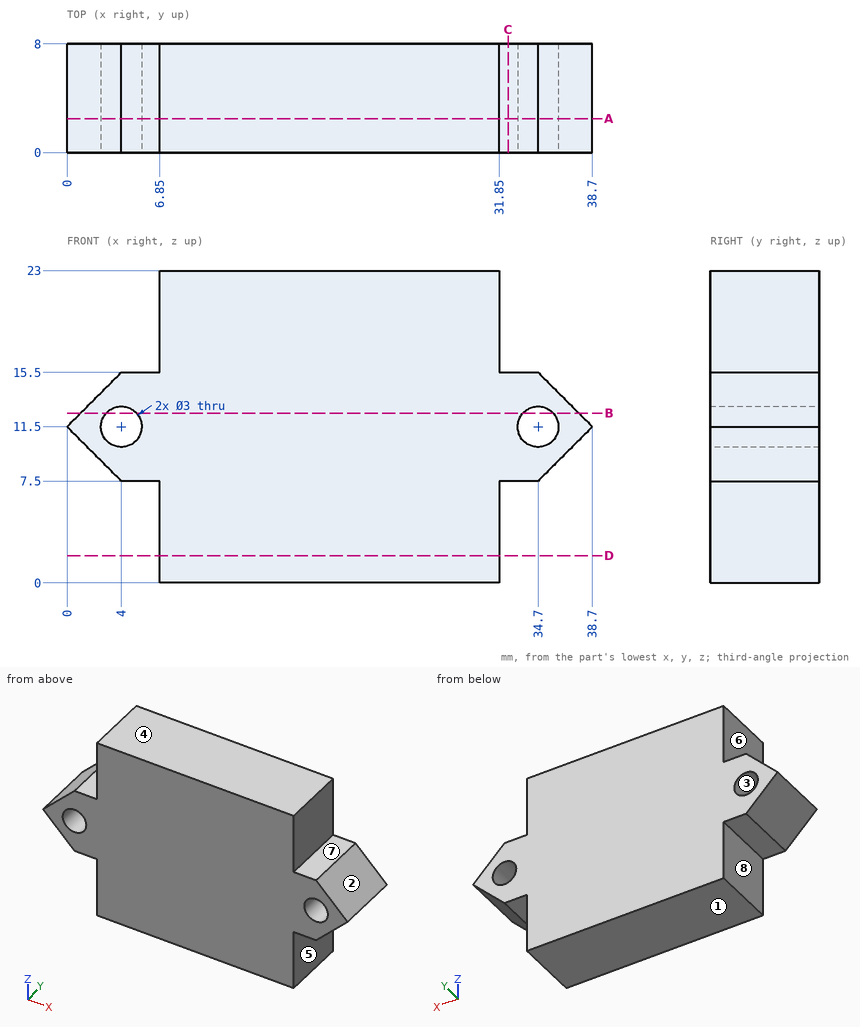
Verification items for this drawing (mm, ordinates from the low corner). A direction names the side the tool comes from. Coordinates: 2 decimals unless noted, no trailing zeros. Loops run counter-clockwise (first coordinate to the right, second up) from the corner with the lowest first, then second, coordinate; pieces in that order, holes last. Notation, with made-up numbers: (-12, 53) -> (37, 53) arc R34 cw to (37, 88) -> close; hole circle Ø8 at (2.25, 11.25). An arc over 180 degrees is marked (long way). Answer in a Markdown table with one row per item. Add a question column.
1. Section check C-C, the plane x = 32.5. Enter the section's corners in (y, z).
2. Section check D-D, the plane z = 2. Enter the section's corners in (x, y), then the cut area to 3 significant figures.
3. Section check B-B, the plane z = 12.5. Enter the section's corners in (x, y).
4. Draft check along Z on the marked faces 1, 2 and 3. Enter one of: +Z half, -Z half, draft (parallel to the pull), parting line (faces both ways), or undercut.
5. Section check A-A, the plane y = 2.5. Enter the section's corners in (x, z).
6. Depth check by flat-ended pin: P1, Ø1, axis at x = 33, y = 4.5, coming from the +Z side; P2, Ø2, axis at y = 3, z = 2.5, coming from the +X side; P3, Ø2.5, axis at x = 5, y = 3.5, coming from the -Z side; P4, Ø2.5, axis at x = 4, z = 11.5, coming from the +Y side. Enter the tip coordinate at first touch or a pass-through.
7. Access from +Z, -Z, +X, -X, +Y, -Y to the whole of each face (thin tool, end or side, straight path). Record for the marked faces 4, 5, 6, 7 and 8.
8. Material ranges on probe 1 along X at (y, z) = (6.25, 10.75); probe 2 along X at (y, z) = (6.25, 7.25); probe 3 along X at (y, z) = (2.25, 9.25), recorded low to high. Write a range as [from, to].
Derived:
| question | item | result |
|---|---|---|
| 1 | outline | (0, 7.5) -> (8, 7.5) -> (8, 15.5) -> (0, 15.5) -> close |
| 2 | outline | (6.85, 0) -> (31.85, 0) -> (31.85, 8) -> (6.85, 8) -> close |
| 2 | area | 200 mm² |
| 3 | outline | (1, 0) -> (2.88, 0) -> (2.88, 8) -> (1, 8) -> close; (5.12, 0) -> (33.58, 0) -> (33.58, 8) -> (5.12, 8) -> close; (35.82, 0) -> (37.7, 0) -> (37.7, 8) -> (35.82, 8) -> close |
| 4 | face 1 | -Z half |
| 4 | face 2 | +Z half |
| 4 | face 3 | undercut |
| 5 | outline | (0, 11.5) -> (4, 7.5) -> (6.85, 7.5) -> (6.85, 0) -> (31.85, 0) -> (31.85, 7.5) -> (34.7, 7.5) -> (38.7, 11.5) -> (34.7, 15.5) -> (31.85, 15.5) -> (31.85, 23) -> (6.85, 23) -> (6.85, 15.5) -> (4, 15.5) -> close; hole circle Ø3 at (4, 11.5); hole circle Ø3 at (34.7, 11.5) |
| 6 | P1 | stops at z = 15.5 |
| 6 | P2 | stops at x = 31.85 |
| 6 | P3 | stops at z = 7.5 |
| 6 | P4 | passes through |
| 7 | face 4 | +Z, +X, -X, +Y, -Y |
| 7 | face 5 | -Z, +X, +Y, -Y |
| 7 | face 6 | +Z, -X, +Y, -Y |
| 7 | face 7 | +Z, +X, +Y, -Y |
| 7 | face 8 | -Z, -X, +Y, -Y |
| 8 | probe 1 | x = [0.75, 2.7], [5.3, 33.4], [36, 37.95] |
| 8 | probe 2 | x = [6.85, 31.85] |
| 8 | probe 3 | x = [2.25, 36.45] |
